Autodesk Inventor part; units mm, degrees
ref_plane "YZ Plane" through (0, 0, 0) normal (1, 0, 0) x (0, 1, 0)
ref_plane "XZ Plane" through (0, 0, 0) normal (0, 1, 0) x (-1, 0, 0)
ref_plane "XY Plane" through (0, 0, 0) normal (0, 0, 1) x (1, 0, 0)
sketch "Sketch1" plane through (0, 0, 0) normal (0, 1, 0) x (-1, 0, 0)
  line L0 (18.6817, 11.7856) -> (-18.6817, 11.7856)
  line L1 (-18.6817, 11.7856) -> (-18.6817, -11.7856)
  line L2 (-18.6817, -11.7856) -> (18.6817, -11.7856)
  line L3 (18.6817, -11.7856) -> (18.6817, 11.7856)
  line L4 (18.6817, 11.7856) -> (-18.6817, -11.7856) construction
  line L5 (-18.6817, 11.7856) -> (18.6817, -11.7856) construction
  point P0 (0, 0)
  dimension "d0" = 37.3634
  dimension "d1" = 23.5712
extrude "Extrusion1" add sketch "Sketch1" against normal blind 8.255
sketch "Sketch2" plane through (0, 0, 0) normal (0, 1, 0) x (1, 0, 0)
  line L0 (-13.6017, -6.7056) -> (13.6017, -6.7056)
  line L1 (13.6017, -6.7056) -> (13.6017, 6.7056)
  line L2 (13.6017, 6.7056) -> (-13.6017, 6.7056)
  line L3 (-13.6017, 6.7056) -> (-13.6017, -6.7056)
  line L4 (-13.6017, -6.7056) -> (13.6017, 6.7056) construction
  line L5 (13.6017, -6.7056) -> (-13.6017, 6.7056) construction
  point P0 (0, 0)
  dimension "d4" = 13.4112
  dimension "d5" = 27.2034
extrude "Extrusion2" cut sketch "Sketch2" against normal blind 1.6002
sketch "Sketch3" plane through (0, -8.255, 0) normal (0, -1, 0) x (1, 0, 0)
  line L0 (10.4521, 3.556) -> (-10.4521, 3.556) construction
  line L1 (-10.4521, 3.556) -> (-10.4521, -3.556) construction
  line L2 (-10.4521, -3.556) -> (10.4521, -3.556) construction
  line L3 (10.4521, -3.556) -> (10.4521, 3.556) construction
  line L4 (10.4521, 3.556) -> (-10.4521, -3.556) construction
  line L5 (-10.4521, 3.556) -> (10.4521, -3.556) construction
  point P0 (0, 0)
  dimension "d8" = 7.112
  dimension "d9" = 20.9042
hole "Hole2" at (10.4521, -8.255, -3.556) at (-10.4521, -8.255, -3.556) at (-10.4521, -8.255, 3.556) at (10.4521, -8.255, 3.556) direction (0, 1, 0) diameter 5.08 depth 3.175
sketch "Sketch14" plane through (10.4521, -5.08, -3.556) normal (0, -1, 0) x (1, 0, 0)
  circle A0 centre (0, 0) radius 2.54
  circle A1 centre (0, 7.112) radius 2.54
  circle A2 centre (-20.9042, 7.112) radius 2.54
  point P0 (-10.4521, 3.556)
  point P1 (-20.9042, 0)
hole "Hole10" at (10.4521, -5.08, -3.556) at (10.4521, -5.08, 3.556) at (-10.4521, -5.08, 3.556) at (-10.4521, -5.08, -3.556) direction (0, 1, 0) diameter 3.302 end through all
sketch "Sketch9" plane through (-10.4521, -5.08, -3.556) normal (0, -1, 0) x (1, 0, 0)
  point P0 (0, 0)
equation "\"d0\" = PartWidth"
equation "\"d1\" = PartLength"
equation "\"d2\" = BaseHeight"
equation "\"d4\" = CanBaseLength"
equation "\"d5\" = CanBaseWidth"
equation "\"d8\" = HoleLength"
equation "\"d9\" = HoleWidth"
equation "\"d18\" = boltHeadDiam"
equation "\"d23\" = boltHeadHeight"
equation "\"d74\" = boltDiamHole"
equation "\"HoleWidth\" = 20.9042"
equation "\"HoleLength\" = 7.112"
equation "\"BaseOffset\" = 5.08"
equation "\"PartWidth\" = CanBaseWidth + 2 * BaseOffset"
equation "\"PartLength\" = CanBaseLength + 2 * BaseOffset"
equation "\"boardGap\" = 0.508"
equation "\"boltHeadHeight\" = 3.175"
equation "\"boltHeadDiam\" = 5.08"
equation "\"boltDiamHole\" = 3.302"
properties part number "BaseForCanBusConnector"
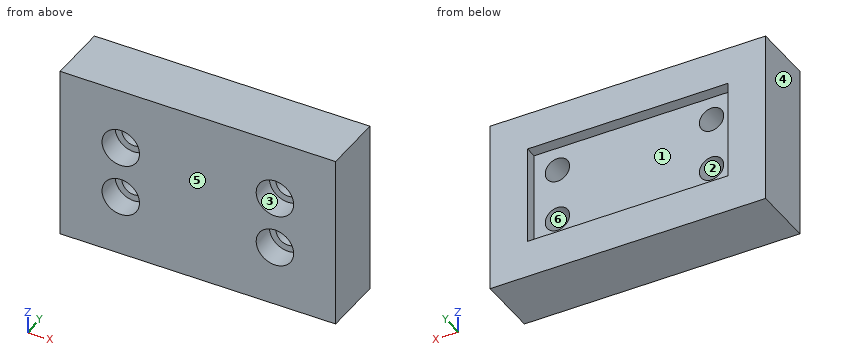
Model file for the job. Use its own axes, mm. Face numbers are marked on the shaded views. A direction names the side the tool comes from. Round coordinates to 2 decimals unless told otherwise and drop trailing zeros. Loops run counter-clockwise (first coordinate to the right, second up) from the corner with the lowest first, then second, coordinate; pieces in that order, holes last.
1. Wall check: probe 1 along X at (y, z) = (-4.75, 3.5); probe 2 along X at (y, z) = (-1.5, 1.75); probe 3 along Z at (x, y) = (0, -0.75). Give the ranges that are in metal, low to high.
Check values:
probe 1: x = -18.68 to -12.1, -8.8 to 8.8, 12.1 to 18.68
probe 2: x = -18.68 to -13.6, 13.6 to 18.68
probe 3: z = -11.79 to -6.71, 6.71 to 11.79
2. Band-saw the part on D-D, the plane y = -6.75. List the corners of the cut face in (x, z), and give its area (3 significant figures).
Check values:
outline: (-18.68, -11.79) - (18.68, -11.79) - (18.68, 11.79) - (-18.68, 11.79) - close; hole circle Ø5.08 at (-10.45, -3.56); hole circle Ø5.08 at (-10.45, 3.56); hole circle Ø5.08 at (10.45, -3.56); hole circle Ø5.08 at (10.45, 3.56)
area: 800 mm2
3. Tool access for the marked faces 1, 2 and 3: list every direction of +Z, -Z, +X, -X, +Y, -Y with a clear straight run to the whole face (end or side of a thin tool).
Check values:
face 1: +Y
face 2: +Y, -Y
face 3: -Y
4. Band-saw the part on C-C, the plane z = 3.75. List the corners of the cut face in (x, y) (3 decimals), and give its area (3 significant figures).
Check values:
outline: (-18.682, -8.255) - (-12.985, -8.255) - (-12.985, -5.08) - (-12.092, -5.08) - (-12.092, -1.6) - (-13.602, -1.6) - (-13.602, 0) - (-18.682, 0) - close; (-8.813, -5.08) - (-7.92, -5.08) - (-7.92, -8.255) - (7.92, -8.255) - (7.92, -5.08) - (8.813, -5.08) - (8.813, -1.6) - (-8.813, -1.6) - close; (12.092, -5.08) - (12.985, -5.08) - (12.985, -8.255) - (18.682, -8.255) - (18.682, 0) - (13.602, 0) - (13.602, -1.6) - (12.092, -1.6) - close
area: 210 mm2
5. Band-saw the part on A-A, the plane y = -1. List the corners of the cut face in (x, z).
Check values:
outline: (-18.68, -11.79) - (18.68, -11.79) - (18.68, 11.79) - (-18.68, 11.79) - close; hole (-13.6, -6.71) - (13.6, -6.71) - (13.6, 6.71) - (-13.6, 6.71) - close
6. Band-saw the part on B-B, the plane x = 1.5. List the corners of the cut face in (y, z) (3 decimals).
Check values:
outline: (-8.255, -11.786) - (0, -11.786) - (0, -6.706) - (-1.6, -6.706) - (-1.6, 6.706) - (0, 6.706) - (0, 11.786) - (-8.255, 11.786) - close
7. Mould opens along X. For the marked faces 4, 5 and 6 say: +X half, -X half, draft (parallel to the pull), parting line (faces both ways), or undercut.
Check values:
face 4: -X half
face 5: draft
face 6: undercut
8. Drop flat-ended pins along their axis: P1, Ø5.5, axis at x = -10.5, z = 2.5, coming from the -Y side (3 decimals); P2, Ø4.5, axis at x = 10.45, z = -3.56, coming from the +Y side; P3, Ø4.5, axis at x = -10.45, z = 3.56, coming from the -Y side. Give the stop position or say it passes through.
Check values:
P1: stops at y = -8.255
P2: stops at y = -1.6
P3: stops at y = -5.08
